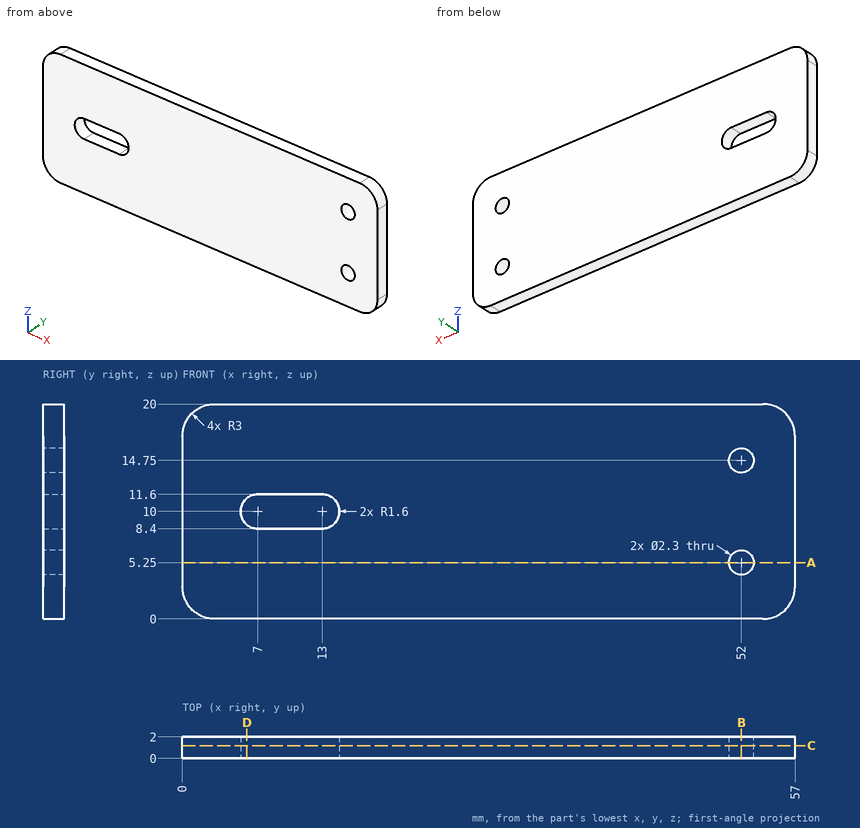
Input: dimensioned drawing with shaded views. Units: mm. Origin: part minimum x, y, z. Coordinates: 2 decimals unless noted, no trailing zeros. Order: outer loops, then holes, each group sorted by start corner. A loop starts at its lowest first (then second) coordinate and runs counter-clockwise, first axis right, second up.
(1) Section query B-B (x = 52). Return the cut outline in (y, z), plus the area to 3 significant figures.
(2) Section query A-A (z = 5.25). Return the cut outline in (x, y), plus the area to 3 significant figures.
(3) Material intervals for probe 1 along Z at (x, y) = (52, 1.4); probe 2 along X at (y, z) = (1.4, 5.25); probe 3 along Z at (x, y) = (53, 0.95), sorted ascending.
(4) First-contact query: pin 1 (1 mm diameter, centred on x = 49.5, y = 1, fed in from -Z). Flat tip, straight axial feed; report the tip coordinate or a pass-through.
(5) Section query C-C (y = 1.2). Return the cut outline in (x, z), plus the area to 3 significant figures.
(6) Section query D-D (x = 6). Return the cut outline in (y, z), plus the area to 3 significant figures.
Solution:
1. outline: (0, 0) - (2, 0) - (2, 4.1) - (0, 4.1) - close; (0, 6.4) - (2, 6.4) - (2, 13.6) - (0, 13.6) - close; (0, 15.9) - (2, 15.9) - (2, 20) - (0, 20) - close
1. area: 30.8 mm2
2. outline: (0, 0) - (50.85, 0) - (50.85, 2) - (0, 2) - close; (53.15, 0) - (57, 0) - (57, 2) - (53.15, 2) - close
2. area: 109 mm2
3. probe 1: z = 0 to 4.1, 6.4 to 13.6, 15.9 to 20
3. probe 2: x = 0 to 50.85, 53.15 to 57
3. probe 3: z = 0 to 4.68, 5.82 to 14.18, 15.32 to 20
4. pin 1: stops at z = 0
5. outline: (0, 3) arc R3 ccw to (3, 0) - (54, 0) arc R3 ccw to (57, 3) - (57, 17) arc R3 ccw to (54, 20) - (3, 20) arc R3 ccw to (0, 17) - close; hole (7, 8.4) - (13, 8.4) arc R1.6 ccw to (13, 11.6) - (7, 11.6) arc R1.6 ccw to start; hole circle Ø2.3 at (52, 5.25); hole circle Ø2.3 at (52, 14.75)
5. area: 1,100 mm2
6. outline: (0, 0) - (2, 0) - (2, 8.75) - (0, 8.75) - close; (0, 11.25) - (2, 11.25) - (2, 20) - (0, 20) - close
6. area: 35.0 mm2
